Can you work these out from the model? Positions are in its coordinate system, mm. A direction names the side the tool comes from. Give positions to 0.01 mm unless a question says otherwise; leave off trailing zeros. Order: outer loops, then holes, each group sorted by start corner. A loop starts at its lowest first (then second) coordinate and runs counter-clockwise, first axis right, second up.
Item 1: I want a section at B-B, the plane y = -101. Write out the boundary of the cut face in (x, z), then the cut area to 3 significant figures.
Item 2: If we mould it in two halves opening along Y, with no side actions, what happens to faces 6 (the cylindrical face through (-249.8, -169.6, 25)), 7 (the cylindrical face through (-182.18, -283.69, 12.12)), 8 (the flat face through (6, -226, 20))? For each: +Y half, -Y half, draft (parallel to the pull), parting line (faces both ways), or undercut.
Item 3: I want a section at A-A, the plane x = -106. Write out the boundary of the cut face in (y, z), then the cut area to 3 significant figures.
Item 4: Which directions (+Z, -Z, +X, -X, +Y, -Y) give clear straight access to the entire face, cutting with the end or side of a thin tool? Please do faces 1 (the cylindrical face through (-57.82, -283.69, 12.12)), 2 (the flat face through (-20, 20.516, 13)), 3 (the flat face through (-225, 20.516, 13)), 4 (the flat face through (-19, -279.484, 13)), 5 (the flat face through (-126, -128, 12)).
Item 5: I'm going to push flat-ended pins straight in: pin 1 Ø2.5 at (x, y) = (14.5, -30) entering from -Z; pin 2 Ø3 at (x, z) = (-83.5, 19) entering from -Y; pin 3 Ø13.5 at (x, y) = (-250.5, -201.5) entering from +Z; pin 4 Ø22 at (x, y) = (-16, 17) entering from +Z. Where does each tip first touch, or does it pass through?
Item 6: If I drill on line 1 along X through (y, z) = (-0.5, 3); line 2 along Y through (x, z) = (-175, 2.5); line 3 along Y through (x, z) = (-134.5, 7), over which ranges is the centre line in solid material (lowest first)?
```python
from build123d import *

# Parameters (mm, degrees)
BOSS_EXTRUDE1_DEPTH  = 5
BOSS_EXTRUDE2_DEPTH  = 15
BOSS_EXTRUDE3_DEPTH  = 10
FILLET1_R            = 5
BOSS_EXTRUDE7_DEPTH  = 10
BOSS_EXTRUDE8_DEPTH  = 10
BOSS_EXTRUDE9_DEPTH  = 10
FILLET5_R            = 5
BOSS_EXTRUDE10_DEPTH = 300
BOSS_EXTRUDE12_DEPTH = 50
BOSS_EXTRUDE13_START = -50
BOSS_EXTRUDE13_DEPTH = 50
CUT_EXTRUDE1_DEPTH   = 12
FILLET7_R            = 5
FILLET8_R            = 3
SKETCH17_W           = 10
SKETCH17_H           = 320
CUT_EXTRUDE2_DEPTH   = 10
FILLET9_R            = 5
SKETCH18_R           = 2.5
CUT_EXTRUDE3_DEPTH   = 10


with BuildPart() as part:
    # Sketch1 → Boss-Extrude1 (new body)
    with BuildSketch(Plane.XY):
        with BuildLine():
            Line((-274.292008101, 30.516404424), (25.707991899, 30.516404424))
            ThreePointArc((25.707991899, 30.516404424), (32.779059711, 27.587472236), (35.707991899, 20.516404424))
            Line((35.707991899, 20.516404424), (35.707991899, -279.483595576))
            ThreePointArc((35.707991899, -279.483595576), (32.779059711, -286.554663388), (25.707991899, -289.483595576))
            Line((25.707991899, -289.483595576), (-274.292008101, -289.483595576))
            ThreePointArc((-274.292008101, -289.483595576), (-281.363075913, -286.554663388), (-284.292008101, -279.483595576))
            Line((-284.292008101, -279.483595576), (-284.292008101, 20.516404424))
            ThreePointArc((-284.292008101, 20.516404424), (-281.363075913, 27.587472236), (-274.292008101, 30.516404424))
        make_face()
    extrude(amount=BOSS_EXTRUDE1_DEPTH)

    # Sketch2 → Boss-Extrude2 (add)
    with BuildSketch(Plane.XY.offset(5)):
        with BuildLine():
            Line((-264.292008101, 20.516404424), (15.707991899, 20.516404424))
            ThreePointArc((15.707991899, 20.516404424), (22.779059711, 17.587472236), (25.707991899, 10.516404424))
            Line((25.707991899, 10.516404424), (25.707991899, -269.483595576))
            ThreePointArc((25.707991899, -269.483595576), (22.779059711, -276.554663388), (15.707991899, -279.483595576))
            Line((15.707991899, -279.483595576), (-264.292008101, -279.483595576))
            ThreePointArc((-264.292008101, -279.483595576), (-271.363075913, -276.554663388), (-274.292008101, -269.483595576))
            Line((-274.292008101, -269.483595576), (-274.292008101, 10.516404424))
            ThreePointArc((-274.292008101, 10.516404424), (-271.363075913, 17.587472236), (-264.292008101, 20.516404424))
        make_face()
    extrude(amount=BOSS_EXTRUDE2_DEPTH)

    # Sketch3 → Boss-Extrude3 (add)
    with BuildSketch(Plane(origin=(-60, 0, 0), x_dir=(0, 0, -1), z_dir=(1, 0, 0))):
        Polygon((-20, 20.516404424), (-5, 20.516404424), (-5, 30.516404424), align=None)
    extrude(amount=BOSS_EXTRUDE3_DEPTH)

    # Fillet1
    fillet1_edges = [part.edges().sort_by_distance(p)[0] for p in [
        (-60, 25.516404424, 12.5),
        (-50, 25.516404424, 12.5),
    ]]
    fillet(fillet1_edges, radius=FILLET1_R - 0.0001)  # a hair under: the kernel refuses the full size

    # Sketch4 → Boss-Extrude7 (add)
    with BuildSketch(Plane(origin=(-180, 0, 0), x_dir=(0, 0, -1), z_dir=(1, 0, 0))):
        Polygon((-20, 20.516404424), (-5, 20.516404424), (-5, 30.516404424), align=None)
    extrude(amount=-BOSS_EXTRUDE7_DEPTH)

    # Sketch9 → Boss-Extrude8 (add)
    with BuildSketch(Plane(origin=(-180, 0, 0), x_dir=(0, 0, -1), z_dir=(1, 0, 0))):
        Polygon((-20, -279.483595576), (-5, -279.483595576), (-5, -289.483595576), align=None)
    extrude(amount=-BOSS_EXTRUDE8_DEPTH)

    # Sketch10 → Boss-Extrude9 (add)
    with BuildSketch(Plane(origin=(-60, 0, 0), x_dir=(0, 0, -1), z_dir=(1, 0, 0))):
        Polygon((-20, -279.483595576), (-5, -279.483595576), (-5, -289.483595576), align=None)
    extrude(amount=BOSS_EXTRUDE9_DEPTH)

    # Fillet5
    fillet5_edges = [part.edges().sort_by_distance(p)[0] for p in [
        (-60, -284.483595576, 12.5),
        (-50, -284.483595576, 12.5),
        (-190, 25.516404424, 12.5),
        (-180, 25.516404424, 12.5),
        (-190, -284.483595576, 12.5),
        (-180, -284.483595576, 12.5),
    ]]
    fillet(fillet5_edges, radius=FILLET5_R - 0.0001)  # a hair under: the kernel refuses the full size

    # Sketch12 → Boss-Extrude10 (add)
    with BuildSketch(Plane.XZ.offset(279.483595576)):
        with BuildLine():
            Line((-229.64600405, 20), (-219.64600405, 20))
            ThreePointArc((-219.64600405, 20), (-224.64600405, 25), (-229.64600405, 20))
        make_face()
        with BuildLine():
            Line((-24.64600405, 20), (-14.64600405, 20))
            ThreePointArc((-14.64600405, 20), (-19.64600405, 25), (-24.64600405, 20))
        make_face()
    extrude(amount=-BOSS_EXTRUDE10_DEPTH)

    # Sketch13 → Boss-Extrude12 (add)
    with BuildSketch(Plane.ZY.offset(274.292008101)):
        with BuildLine():
            Line((20, -84.483595576), (20, -94.483595576))
            ThreePointArc((20, -94.483595576), (25, -89.483595576), (20, -84.483595576))
        make_face()
        with BuildLine():
            Line((20, -164.483595576), (20, -174.483595576))
            ThreePointArc((20, -174.483595576), (25, -169.483595576), (20, -164.483595576))
        make_face()
    extrude(amount=-BOSS_EXTRUDE12_DEPTH)

    # Sketch15 → Boss-Extrude13 (add)
    with BuildSketch(Plane(origin=(25.707991899, 0, 0), x_dir=(0, 0, -1), z_dir=(1, 0, 0)).offset(BOSS_EXTRUDE13_START)):
        with BuildLine():
            Line((-20, -84.483595576), (-20, -94.483595576))
            ThreePointArc((-20, -94.483595576), (-25, -89.483595576), (-20, -84.483595576))
        make_face()
        with BuildLine():
            Line((-20, -164.483595576), (-20, -174.483595576))
            ThreePointArc((-20, -174.483595576), (-25, -169.483595576), (-20, -164.483595576))
        make_face()
    extrude(amount=BOSS_EXTRUDE13_DEPTH)

    # Sketch16 → Cut-Extrude1 (cut)
    with BuildSketch(Plane(origin=(0, 0, 0), x_dir=(-1, 0, 0), z_dir=(0, 0, -1))):
        Polygon((14.292008101, 10.516404424), (264.292008101, 10.516404424), (264.292008101, -269.483595576), (14.292008101, -269.483595576), (14.292008101, -189.483595576), (-15.707991899, -189.483595576), (-15.707991899, -69.483595576), (14.292008101, -69.483595576), align=None)
    extrude(amount=-CUT_EXTRUDE1_DEPTH, mode=Mode.SUBTRACT)

    # Fillet7
    fillet7_edges = [part.edges().sort_by_distance(p)[0] for p in [
        (-14.292008101, -69.483595576, 6),
        (-14.292008101, 10.516404424, 6),
        (-264.292008101, 10.516404424, 6),
        (-264.292008101, -269.483595576, 6),
        (-14.292008101, -269.483595576, 6),
        (-14.292008101, -189.483595576, 6),
        (15.707991899, -189.483595576, 6),
        (15.707991899, -69.483595576, 6),
    ]]
    fillet(fillet7_edges, radius=FILLET7_R)

    # Fillet8
    fillet8_edges = [part.edges().sort_by_distance(p)[0] for p in [
        (-264.292008101, -129.483595576, 12),
        (-139.292008101, -269.483595576, 12),
        (-14.292008101, -29.483595576, 12),
        (0.707991899, -69.483595576, 12),
        (15.707991899, -129.483595576, 12),
        (0.707991899, -189.483595576, 12),
        (-14.292008101, -229.483595576, 12),
        (-139.292008101, 10.516404424, 12),
        (-262.827542007, 9.05193833, 12),
        (-15.756474195, 9.05193833, 12),
        (14.243525805, -70.94806167, 12),
        (14.243525805, -188.019129482, 12),
        (-15.756474195, -268.019129482, 12),
        (-262.827542007, -268.019129482, 12),
        (-12.827542007, -190.94806167, 12),
        (-12.827542007, -68.019129482, 12),
    ]]
    fillet(fillet8_edges, radius=FILLET8_R)

    # Sketch17 → Cut-Extrude2 (cut)
    with BuildSketch(Plane(origin=(0, 0, 0), x_dir=(-1, 0, 0), z_dir=(0, 0, -1))):
        with Locations((-30.707991899, -129.483595576)):
            Rectangle(SKETCH17_W, SKETCH17_H)
    extrude(amount=-CUT_EXTRUDE2_DEPTH, mode=Mode.SUBTRACT)

    # Fillet9
    fillet9_edges = [part.edges().sort_by_distance(p)[0] for p in [
        (25.707991899, -289.483595576, 2.5),
        (25.707991899, 30.516404424, 2.5),
    ]]
    fillet(fillet9_edges, radius=FILLET9_R)

    # Sketch18 → Cut-Extrude3 (cut)
    with BuildSketch(Plane(origin=(0, 0, 0), x_dir=(-1, 0, 0), z_dir=(0, 0, -1))):
        with Locations((4.292008101, -4.483595576)):
            Circle(SKETCH18_R)
        with Locations((-15.507991899, -29.483595576)):
            Circle(SKETCH18_R)
        with Locations((4.292008101, -54.483595576)):
            Circle(SKETCH18_R)
        with Locations((4.292008101, -204.483595576)):
            Circle(SKETCH18_R)
        with Locations((-13.25844967, -229.483595576)):
            Circle(SKETCH18_R)
        with Locations((4.292008101, -254.483595576)):
            Circle(SKETCH18_R)
    extrude(amount=-CUT_EXTRUDE3_DEPTH, mode=Mode.SUBTRACT)


solid = part.part
```
Results list:
1. outline: (-284.29, 0) - (-264.29, 0) - (-264.29, 9) arc R3 cw to (-261.29, 12) - (12.71, 12) arc R3 cw to (15.71, 9) - (15.71, 0) - (25.71, 0) - (25.71, 20) - (-14.65, 20) arc R5 ccw to (-24.65, 20) - (-219.65, 20) arc R5 ccw to (-229.65, 20) - (-274.29, 20) - (-274.29, 5) - (-284.29, 5) - close
1. area: 2,770 mm2
2. face 6: undercut
2. face 7: -Y half
2. face 8: draft
3. outline: (-289.48, 0) - (-269.48, 0) - (-269.48, 9) arc R3 cw to (-266.48, 12) - (7.52, 12) arc R3 cw to (10.52, 9) - (10.52, 0) - (30.52, 0) - (30.52, 5) - (20.52, 5) - (20.52, 20) - (-279.48, 20) - (-279.48, 5) - (-289.48, 5) - close
3. area: 2,740 mm2
4. face 1: +Z, -Y
4. face 2: +Z, +X, +Y
4. face 3: +Z, -X, +Y
4. face 4: +Z, +X, -Y
4. face 5: -Z
5. pin 1: stops at z = 10
5. pin 2: stops at y = -279.48
5. pin 3: stops at z = 20
5. pin 4: stops at z = 25
6. line 1: x = -284.29 to -264.29, -14.29 to 25.71
6. line 2: y = -289.48 to -269.48, 10.52 to 30.52
6. line 3: y = -279.48 to -269.48, 10.52 to 20.52
